Read the model definition and answer for the solid it produces. Units are mm, in the model's axes. A direction names the side the tool comes from. Coordinates: 2 decimals unless noted, no trailing zeros. Loops run counter-clockwise (first coordinate to the right, second up) from the corner with the lowest first, then second, coordinate; pieces in that order, holes last. Notation, with made-up numbers: M -15,69 L 22,69 A12 ccw 22,87 Z; hole C 58.5,-4.75 d5. An arc over 180 degrees is marked long. One line per item, written item: value. Start each with the question number.
1. The part is cut by section A-A (z = 0). Write down the section's boundary in (x, y).
2. The part is cut by section B-B (y = 0.2). Write down the section's boundary in (x, z), then the cut area to 3 significant figures.
3. The part is cut by section D-D (z = 7.75). Write down the section's boundary in (x, y).
4. A flat-ended cylindrical pin translates along its axis: pin 1 (0.5 mm diameter, centred on x = -1.5, y = 0.5, fed in from -Z). Find the tip coordinate at first contact, or state that the pin passes through.
5. Consider probe 1 along Z at (x, y) = (2.5, 0.9); probe 2 along X at (y, z) = (0.1, 2.5); probe 3 along Z at (x, y) = (-1.25, 0.7). Determine where each line is inside the solid, lowest interval first.
6. For faces 1 (the face through (5, 1, 0)), 2 (the face through (-4.25, 0.5, 0.1)), determine the directions among +Z, -Z, +X, -X, +Y, -Y from which every point of the face is accessible in a straight line to the end or side of a thin tool.
7. Determine the mould class of faces 3 (the face through (8.3, 0.5, -9.5)), 4 (the face through (5, 0, 0)), 5 (the face through (-0.1, 0.5, -4.25)), 6 (the face through (19, 0.5, 0.1)) for opening direction Z: +Z half, -Z half, draft (parallel to the pull), parting line (faces both ways), or undercut.
8. The part is cut by section C-C (x = 0.5). Write down the section's boundary in (y, z).
```python
from build123d import *

# Parameters (mm, degrees)
SKIZZE1_W                       = 8.5
SKIZZE1_H                       = 8.5
AUFSATZ_LINEAR_AUSTRAGEN1_DEPTH = 1


with BuildPart() as part:
    # Skizze1 → Aufsatz-Linear austragen1 (new body)
    with BuildSketch(Plane(origin=(0, 0, 0), x_dir=(1, 0, 0), z_dir=(0, 1, 0))):
        with BuildLine():
            Line((0, -9.5), (16.454482672, -9.5))
            ThreePointArc((16.454482672, -9.5), (19, 0), (16.454482672, 9.5))
            Line((16.454482672, 9.5), (0, 9.5))
            ThreePointArc((0, 9.5), (-9.5, 0), (0, -9.5))
        make_face()
        Rectangle(SKIZZE1_W, SKIZZE1_H, mode=Mode.SUBTRACT)
    extrude(amount=AUFSATZ_LINEAR_AUSTRAGEN1_DEPTH)


solid = part.part
```
Answer block:
1. outline: M -9.5,0 L -4.25,0 L -4.25,1 L -9.5,1 Z; M 4.25,0 L 19,0 L 19,1 L 4.25,1 Z
2. outline: M 0,-9.5 L 16.45,-9.5 A19 ccw 16.45,9.5 L 0,9.5 A9.5 ccw Z; hole M -4.25,-4.25 L 4.25,-4.25 L 4.25,4.25 L -4.25,4.25 Z
2. area: 415 mm2
3. outline: M -5.49,0 L 17.35,0 L 17.35,1 L -5.49,1 Z
4. pin 1: stops at z = -9.42
5. probe 1: z = -9.5 to -4.25, 4.25 to 9.5
5. probe 2: x = -9.17 to -4.25, 4.25 to 18.83
5. probe 3: z = -9.42 to -4.25, 4.25 to 9.42
6. face 1: +Z, -Z, +X, -X, +Y
6. face 2: +Y, -Y
7. face 3: -Z half
7. face 4: draft
7. face 5: undercut
7. face 6: parting line
8. outline: M 0,-9.5 L 1,-9.5 L 1,-4.25 L 0,-4.25 Z; M 0,4.25 L 1,4.25 L 1,9.5 L 0,9.5 Z
